Read the model definition and answer for the solid it produces. Units are mm, in the model's axes. Coordinates: 2 decimals unless noted, no trailing zeros. Loops run counter-clockwise (first coordinate to the right, second up) from the corner with the lowest first, then second, coordinate; pieces in that order, holes last. Notation, with made-up numbers: (-23.5, 29) -> (2.5, 29) arc R21 ccw to (2.5, 64) -> close; hole circle Ø7 at (49.5, 63.25). An arc over 180 degrees is marked (long way). Answer as a JSON object with one key per item and string values. Group by question number.
Q1. A straight line is drawn through the part: line 1 along Y through (x, z) = (2.75, -401.5). Find the intervals that lie inside material, in ascending order. Write a range as [from, to].
Q2. The part is cut by section A-A on x = 3. Write down the section's boundary in (y, z), and give its area (3 significant figures).
Q3. Each of these flat-tipped pins is pushed along its axis until it touches: P1, Ø1.9, axis at x = 3.5, y = 3.5, coming from the +Z side; P2, Ø1.9, axis at x = 2, z = -168.5, coming from the -Y side; P3, Ø1.9, axis at x = 4, y = 2.5, coming from the -Z side. Where does it stop, or does it pass through?
Q4. The part is cut by section B-B on z = -97. Write down the section's boundary in (x, y).
from build123d import *

# Parameters (mm, degrees)
SKETCH1_W           = 435
SKETCH1_H           = 31.75
BOSS_EXTRUDE1_DEPTH = 6.35
CUT_EXTRUDE1_REACH  = 441.326
SKETCH2_W           = 101.6
SKETCH2_H           = 6.35
CUT_EXTRUDE2_REACH  = 441.326
SKETCH3_W           = 50.8
SKETCH3_H           = 6.35
SKETCH3_W_2         = 79.4


with BuildPart() as part:
    # Sketch1 → Boss-Extrude1 (new body)
    with BuildSketch(Plane(origin=(0, 0, 0), x_dir=(0, 0, -1), z_dir=(1, 0, 0))):
        with Locations((220.631015664, 15.875)):
            Rectangle(SKETCH1_W, SKETCH1_H)
    extrude(amount=BOSS_EXTRUDE1_DEPTH)

    # Sketch2 → Cut-Extrude1 (cut, up to next)
    with BuildSketch(Plane.ZY, mode=Mode.PRIVATE) as cut_extrude1_sk1:
        with Locations((-53.931015664, 3.175)):
            Rectangle(SKETCH2_W, SKETCH2_H)
    cut_extrude1_tool1 = extrude(cut_extrude1_sk1.sketch, amount=-CUT_EXTRUDE1_REACH, mode=Mode.PRIVATE) & part.part
    add(cut_extrude1_tool1.solids().sort_by_distance((0, 3.175, -53.931016))[0], mode=Mode.SUBTRACT)

    # Sketch3 → Cut-Extrude2 (cut, up to next)
    with BuildSketch(Plane.ZY, mode=Mode.PRIVATE) as cut_extrude2_sk1:
        with Locations((-180.931015664, 3.175)):
            Rectangle(SKETCH3_W, SKETCH3_H)
    cut_extrude2_tool1 = extrude(cut_extrude2_sk1.sketch, amount=-CUT_EXTRUDE2_REACH, mode=Mode.PRIVATE) & part.part
    # Sketch3 → Cut-Extrude2 (cut, up to next)
    with BuildSketch(Plane.ZY, mode=Mode.PRIVATE) as cut_extrude2_sk2:
        with Locations((-282.531015664, 3.175)):
            Rectangle(SKETCH3_W, SKETCH3_H)
    cut_extrude2_tool2 = extrude(cut_extrude2_sk2.sketch, amount=-CUT_EXTRUDE2_REACH, mode=Mode.PRIVATE) & part.part
    # Sketch3 → Cut-Extrude2 (cut, up to next)
    with BuildSketch(Plane.ZY, mode=Mode.PRIVATE) as cut_extrude2_sk3:
        with Locations((-398.431015664, 3.175)):
            Rectangle(SKETCH3_W_2, SKETCH3_H)
    cut_extrude2_tool3 = extrude(cut_extrude2_sk3.sketch, amount=-CUT_EXTRUDE2_REACH, mode=Mode.PRIVATE) & part.part
    add(cut_extrude2_tool1.solids().sort_by_distance((0, 3.175, -180.931016))[0], mode=Mode.SUBTRACT)
    add(cut_extrude2_tool2.solids().sort_by_distance((0, 3.175, -282.531016))[0], mode=Mode.SUBTRACT)
    add(cut_extrude2_tool3.solids().sort_by_distance((0, 3.175, -398.431016))[0], mode=Mode.SUBTRACT)


solid = part.part
Final values:
{
 "1": {"line 1": "y = [6.35, 31.75]"},
 "2": {"outline": "(0, -358.73) -> (6.35, -358.73) -> (6.35, -438.13) -> (31.75, -438.13) -> (31.75, -3.13) -> (6.35, -3.13) -> (6.35, -104.73) -> (0, -104.73) -> (0, -155.53) -> (6.35, -155.53) -> (6.35, -206.33) -> (0, -206.33) -> (0, -257.13) -> (6.35, -257.13) -> (6.35, -307.93) -> (0, -307.93) -> close", "area": "12,000 mm2"},
 "3": {"P1": "stops at z = -104.73", "P2": "stops at y = 6.35", "P3": "stops at z = -358.73"},
 "4": {"outline": "(0, 6.35) -> (6.35, 6.35) -> (6.35, 31.75) -> (0, 31.75) -> close"}
}
